The model under review builds one solid part; all positions refer to its coordinate system, in mm. Face numbers are marked on the shaded views. Round coordinates to 2 decimals unless told otherwise and drop trailing zeros. Loops run counter-clockwise (first coordinate to the right, second up) from the corner with the lowest first, then second, coordinate; pieces in that order, holes last. Notation, with made-up numbers: (86, 20) - (137, 20) arc R19 cw to (137, 46) - close; hole circle Ø11 at (80.25, -37.5). An arc over 180 degrees is marked (long way). Answer as CSV lines item,"result".
Autodesk Inventor part; units mm, degrees
ref_plane "YZ Plane" through (0, 0, 0) normal (1, 0, 0) x (0, 1, 0)
ref_plane "XZ Plane" through (0, 0, 0) normal (0, 1, 0) x (-1, 0, 0)
ref_plane "XY Plane" through (0, 0, 0) normal (0, 0, 1) x (1, 0, 0)
sketch "Sketch1" plane through (0, 0, 0) normal (0, 0, 1) x (1, 0, 0)
  circle A0 centre (-152.5842, 1.6449) radius 20
  circle A1 centre (-2.5848, 1.2498) radius 20
  arc A2 (-157.1373, 21.1198) -> (-0.3077, 21.1198) centre (-78.7225, 413.3584) ccw
  arc A3 (3.2676, -17.8748) -> (-158.9335, -17.3205) centre (-79.1716, -409.2873) ccw
  dimension "d5" = 40
  dimension "d6" = 40
  dimension "d7" = 150
  dimension "d8" = 400
  dimension "d9" = 400
extrude "Extrusion1" add sketch "Sketch1" along normal blind 4 contours A2 A0 A3 | A2 A1 A3 A0 | A2 A1 A3
sketch "Sketch2" plane through (0, 0, 4) normal (0, 0, 1) x (1, 0, 0)
  arc A0 (-157.1373, 21.1198) -> (-158.9335, -17.3205) centre (-152.5842, 1.6449) ccw
  circle A1 centre (-152.5842, 1.6449) radius 4
  point P0 (0, 0)
  dimension "d12" = 8
extrude "Extrusion2" add sketch "Sketch2" along normal blind 11.9
sketch "Sketch3" plane through (-152.5842, 1.6449, 15.9) normal (0, 0, 1) x (1, 0, 0)
  circle A0 centre (0, 0) radius 2.75
  point P0 (152.5842, -1.6449)
  dimension "d16" = 5.5
extrude "Extrusion3" cut sketch "Sketch3" against normal blind 5
sketch "Sketch4" plane through (0, 0, 0) normal (0, 0, -1) x (-1, 0, 0)
  arc A0 (0.3077, 21.1198) -> (-3.2676, -17.8748) centre (2.5848, 1.2498) ccw
  line L0 (0.3077, 21.1198) -> (0.3077, -17.1388)
  arc A1 (158.9335, -17.3205) -> (-3.2676, -17.8748) centre (79.1716, -409.2873) ccw
  point P0 (0, 0)
extrude "Extrusion4" add sketch "Sketch4" along normal blind 15 and the other way blind 19
sketch "Sketch5" plane through (0, 0, -15) normal (0, 0, -1) x (-1, 0, 0)
  arc A0 (0.3077, 21.1198) -> (-3.2676, -17.8748) centre (2.5848, 1.2498) ccw
  line L0 (-3.2676, 20.3744) -> (-3.2676, -17.8748)
  point P0 (0, 0)
extrude "Extrusion5" cut sketch "Sketch5" against normal blind 35
sketch "Sketch6" plane through (-152.5842, 1.6449, 15.9) normal (0, 0, 1) x (1, 0, 0)
  point P0 (152.5842, -1.6449)
sketch "Sketch7" plane through (-0.3077, -17.1388, 4) normal (-1, 0, 0) x (0, 0, 1)
  point P0 (-4, 17.1388)
sketch "Sketch8" plane through (-0.3077, -17.1388, 4) normal (-1, 0, 0) x (0, 0, 1)
  point P0 (-4, 17.1388)
sketch "Sketch9" plane through (3.2676, -17.8748, -15) normal (1, 0, 0) x (0, 0, -1)
  circle A0 centre (-4, 4) radius 1.475
  circle A1 centre (-4, 34.2492) radius 1.475
  circle A2 centre (-30, 4) radius 1.475
  circle A3 centre (-30, 34.2492) radius 1.475
  line L0 (0, 38.2492) -> (0, 0)
  line L1 (-34, 0) -> (-34, 38.2492)
  line L2 (0, 0) -> (-34, 0)
  line L3 (-34, 38.2492) -> (0, 38.2492)
  point P0 (-15, 17.8748)
  dimension "d27" = 2.95
  dimension "d28" = 2.95
  dimension "d29" = 2.95
  dimension "d30" = 2.95
  dimension "d31" = 4
  dimension "d32" = 4
  dimension "d33" = 4
  dimension "d34" = 4
  dimension "d35" = 4
  dimension "d36" = 4
  dimension "d37" = 4
  dimension "d38" = 4
extrude "Extrusion6" cut sketch "Sketch9" against normal blind 5 contours A0 | A1 | A2 | A3
sketch "Sketch10" plane through (0, 0, 4) normal (0, 0, 1) x (1, 0, 0)
  point P0 (0, 0)
sketch "Sketch11" plane through (0, 0, 4) normal (0, 0, 1) x (1, 0, 0)
  point P0 (0, 0)
sketch "Sketch12" plane through (0, 0, 4) normal (0, 0, 1) x (1, 0, 0)
  point P0 (0, 0)
sketch "Sketch13" plane through (0, 0, 4) normal (0, 0, 1) x (1, 0, 0)
  circle A0 centre (-113.0156, 1.6449) radius 10.301
  circle A1 centre (-90.0292, 1.6449) radius 8.912
  circle A2 centre (-66.9339, 1.6449) radius 9.4643
  circle A3 centre (-43.8386, 1.6449) radius 10.301
  circle A4 centre (-21.0701, 1.6449) radius 10.301
  circle A5 centre (-135.3483, 1.6449) radius 9.3403
  point P0 (0, 0)
extrude "Extrusion7" cut sketch "Sketch13" against normal blind 10
sketch "Sketch14" plane through (3.2676, -17.8748, -15) normal (1, 0, 0) x (0, 0, -1)
  line L0 (-17.5, 18.3748) -> (-16.5, 18.3748)
  line L1 (-16.5, 18.3748) -> (-16.5, 17.3748)
  line L2 (-16.5, 17.3748) -> (-17.5, 17.3748)
  line L3 (-17.5, 17.3748) -> (-17.5, 18.3748)
  line L4 (-17.5, 18.3748) -> (-16.5, 17.3748) construction
  line L5 (-16.5, 18.3748) -> (-17.5, 17.3748) construction
  point P0 (-15, 17.8748)
  point P1 (-17, 17.8748)
  dimension "d43" = 1
  dimension "d44" = 1
extrude "Extrusion8" cut sketch "Sketch14" against normal blind 0.1
properties part number "arm" material "Aluminum 6061"
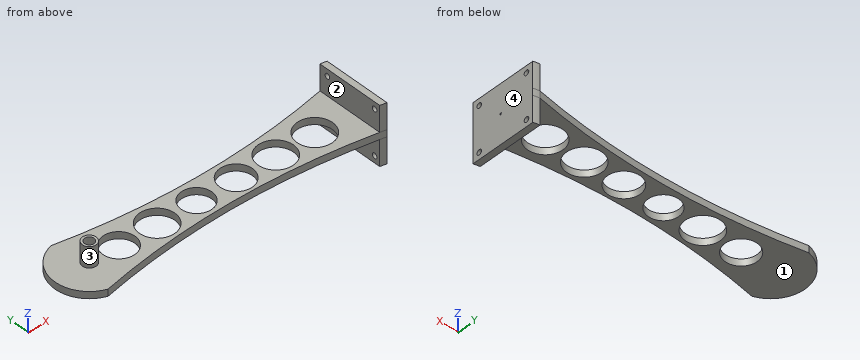
1. Take a section at D-D (z = 5.5). State the section outline as (x, y) points, plus the area to 3 significant figures.
Numbers:
outline,"circle Ø8 at (-152.58, 1.64); (-0.31, -17.14) arc R400 cw to (3.27, -17.87) - (3.27, 20.37) arc R20 ccw to (-0.31, 21.12) - close"
area,"187 mm²"
2. Wall thickness on probe 1 along X at (y, z) = (15, -0.5); probe 2 along Z at (x, y) = (-155, 4.5); probe 3 along Z at (x, y) = (-144.5, -3): over which ranges is each line inside the solid? List them lowest first.
Numbers:
probe 1,"x = -0.31 to 3.27"
probe 2,"z = 0 to 15.9"
probe 3,"z = 0 to 4"
3. Take a section at A-A (y = 8). State how many separate pieces and enclosed holes the cut face has, plus the area to 3 significant figures.
Numbers:
separate pieces,"7"
enclosed holes,"0"
area,"451 mm²"
4. Clearance check with flat-ended pins moving along their axes: pin 1 (12 mm diameter, centred on x = -62.5, z = 14, fed in from -Y); pin 2 (4 mm diameter, centred on x = -128.5, z = -1.5, fed in from +Y); pin 3 (3 mm diameter, centred on y = 4.5, z = -8, fed in from -X); pin 4 (19 mm diameter, centred on x = -112.5, y = 3, fed in from -Z). State where each tip first meets the part, or that it passes through.
Numbers:
pin 1,"passes through"
pin 2,"stops at y = 16.64"
pin 3,"stops at x = -0.31"
pin 4,"stops at z = 0"
5. Take a section at C-C (z = -11). State the section outline as (x, y) points, plus the area to 3 significant figures.
Numbers:
outline,"(-0.31, -17.14) arc R400 cw to (3.27, -17.87) - (3.27, -15.35) - (-0.31, -15.35) - close; (-0.31, -12.4) - (3.27, -12.4) - (3.27, 14.9) - (-0.31, 14.9) - close; (-0.31, 17.85) - (3.27, 17.85) - (3.27, 20.37) arc R20 ccw to (-0.31, 21.12) - close"
area,"116 mm²"
6. Draft analysis for pull direction X (two halves, no side actions). For the marked faces 1, 2, 3 and 4, state which applies: +X half, -X half, draft (parallel to the pull), parting line (faces both ways), or undercut.
Numbers:
face 1,"draft"
face 2,"undercut"
face 3,"undercut"
face 4,"+X half"
